Input: dimensioned drawing with shaded views. Units: mm. Origin: part minimum x, y, z. A direction names the side the tool comes from. Round coordinates to 2 decimals unless told otherwise and drop trailing zeros. Loops run counter-clockwise (first coordinate to the right, second up) from the corner with the lowest first, then second, coordinate; pieces in that order, holes last. Notation, with made-up numbers: (13, 24.25) - (27, 24.25) arc R22 cw to (27, 39.25) - close; hole circle Ø4 at (56, 68). An arc over 180 degrees is marked (long way). Write each question's results on one line, items separated by ' | '.
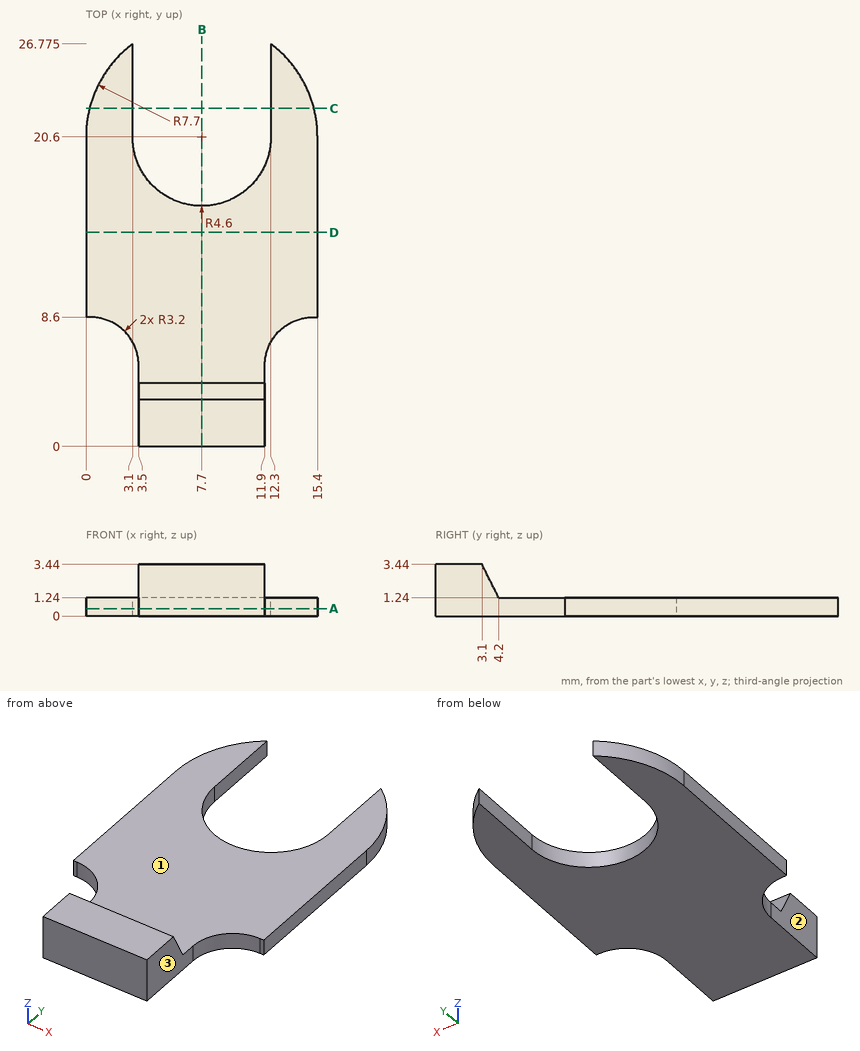
1. Line query: line 1 (X direction, y = 3, z = 0.4); line 2 (X direction, y = 25.5, z = 0.65); line 3 (Z direction, x = 6.5, y = 8.5). Output: solid intervals per line, ascending. Write a range as [from, to].
Answer:
line 1: [3.5, 11.9] | line 2: [1.76, 3.1], [12.3, 13.64] | line 3: [0, 1.24]
2. Section query B-B, the plane x = 7.7. Output: boundary loops of the cut face in (y, z), plus the area to 3 significant figures.
Answer:
outline: (0, 0) - (16, 0) - (16, 1.24) - (4.2, 1.24) - (3.1, 3.44) - (0, 3.44) - close | area: 27.9 mm^2
3. Section query D-D, the plane y = 14.25. Output: boundary loops of the cut face in (x, z).
Answer:
outline: (0, 0) - (15.4, 0) - (15.4, 1.24) - (0, 1.24) - close
4. Set-up query: the marked faces 1, 2 and 3. Return all of +Z, -Z, +X, -X, +Y, -Y with unobstructed straight access to the full face (end or side cutting, diameter ignored); none if empty.
Answer:
face 1: +Z, +X, -X, +Y | face 2: +Z, -Z, -X, -Y | face 3: +Z, -Z, +X, -Y
5. Section query C-C, the plane y = 22.5. Output: boundary loops of the cut face in (x, z), plus the area to 3 significant figures.
Answer:
outline: (0.24, 0) - (3.1, 0) - (3.1, 1.24) - (0.24, 1.24) - close; (12.3, 0) - (15.16, 0) - (15.16, 1.24) - (12.3, 1.24) - close | area: 7.10 mm^2
6. Contact query for flat-ended pins moving along their axis: pin 1 (2 mm diameter, centred on x = 2, z = 2, fed in from +Y); pin 2 (7.5 mm diameter, centred on x = 6.5, y = 18, fed in from +Z); pin 3 (0.6 mm diameter, centred on y = 22.5, z = 1, fed in from -X). Output: stop coordinate, or through.
Answer:
pin 1: y = 26.41 | pin 2: z = 1.24 | pin 3: x = 0.17
7. Section query A-A, the plane z = 0.5. Output: boundary loops of the cut face in (x, y) (3 decimals), plus the area to 3 significant figures.
Answer:
outline: (0, 8.6) - (0.3, 8.6) arc R3.2 cw to (3.5, 5.4) - (3.5, 0) - (11.9, 0) - (11.9, 5.4) arc R3.2 cw to (15.1, 8.6) - (15.4, 8.6) - (15.4, 20.6) arc R7.7 ccw to (12.3, 26.775) - (12.3, 20.6) arc R4.6 cw to (3.1, 20.6) - (3.1, 26.775) arc R7.7 ccw to (0, 20.6) - close | area: 255 mm^2
